Input: part model. Units: mm. Frame: model coordinates. Coordinates: 2 decimals unless noted, no trailing zeros. Write each loop counter-clockwise with the first axis right and the second up, starting at its lowest first coordinate (ties: lowest second). Pieces come first, ordered by that corner, then holes. Notation, with made-up numbers: (27, -23) - (86, -23) arc R22 cw to (86, 0) - close; hole circle Ø6 at (30, 2.25). An arc over 180 degrees is marked (long way). One line per question, with ' | ' between items. Start each with the question number.
1) First-contact query: P1, Ø0.9, axis at y = 15.5, z = 1, coming from the +X side; P2, Ø0.9, axis at y = 27.5, z = 2, coming from the +X side; P3, Ø1.5, axis at y = 25, z = 2, coming from the -X side. Flat tips, straight axial feed; report the tip coordinate or a pass-through.
2) Section query A-A on y = 68.5. Return loops of the section in (x, z), and give its area (3 significant figures).
3) Draft query along X for faces 1 (the cylindrical face through (182.45, 72.19, 1.48)), 2 (the flat face through (140, 15, 0)), 3 (the cylindrical face through (196.41, 57.77, 1.48)). Return one class per face: released by +X, released by -X, zero draft, split by the parting line, or undercut.
4) Section query C-C on x = 105. Return loops of the section in (y, z), and give its area (3 significant figures).
5) Line query: line 1 (Y direction, x = 228.5, z = 0.55); line 2 (Y direction, x = 166.5, z = 1.1); line 3 (X direction, y = 15.5, z = 1.4). Output: solid intervals per line, ascending.
6) Section query D-D on y = 58.5. Return loops of the section in (x, z), and give its area (3 significant figures).
7) Section query B-B on z = 1.15. Return loops of the section in (x, y), and give its area (3 significant figures).
```python
from build123d import *

# Parameters (mm, degrees)
EXTRUDE_1_DEPTH = 3


with BuildPart() as part:
    # Эскиз2 → Бобышка-Вытянуть1 (new body)
    with BuildSketch(Plane.XY):
        with BuildLine():
            Line((0, 0), (172, 0))
            Line((172, 0), (172, 6))
            Line((172, 6), (177, 6))
            Line((177, 6), (177, 0))
            Line((177, 0), (244, 0))
            Line((244, 0), (244, 6))
            Line((244, 6), (250, 6))
            Line((250, 6), (250, 12))
            Line((250, 12), (244, 12))
            Line((244, 12), (214, 12))
            Line((214, 12), (214, 20))
            Line((214, 20), (187, 20))
            Line((187, 20), (187, 32))
            ThreePointArc((187, 32), (196.668498224, 58.076809621), (221, 71.547439867))
            Line((221, 71.547439867), (231, 71.547439867))
            Line((231, 71.547439867), (231, 51.547439867))
            Line((231, 51.547439867), (241, 51.547439867))
            Line((241, 51.547439867), (241, 83.547439867))
            ThreePointArc((241, 83.547439867), (238.656854249, 89.204294116), (233, 91.547439867))
            Line((233, 91.547439867), (219.644566271, 91.547439867))
            ThreePointArc((219.644566271, 91.547439867), (182.048214587, 71.740873017), (167, 32))
            Line((167, 32), (167, 20))
            Line((167, 20), (0, 20))
            Line((0, 20), (-6, 20))
            Line((-6, 20), (-6, 14))
            Line((-6, 14), (0, 14))
            Line((0, 14), (0, 6))
            Line((0, 6), (-6, 6))
            Line((-6, 6), (-6, 0))
            Line((-6, 0), (0, 0))
        make_face()
    extrude(amount=EXTRUDE_1_DEPTH)


solid = part.part
```
Answer key:
1) P1: x = 214 | P2: x = 187 | P3: x = 167
2) outline: (179.38, 0) - (210.64, 0) - (210.64, 3) - (179.38, 3) - close; (231, 0) - (241, 0) - (241, 3) - (231, 3) - close | area: 124 mm²
3) face 1: released by -X | face 2: zero draft | face 3: undercut
4) outline: (0, 0) - (20, 0) - (20, 3) - (0, 3) - close | area: 60.0 mm²
5) line 1: 0 to 12, 71.55 to 91.55 | line 2: 0 to 20 | line 3: -6 to 214
6) outline: (173.17, 0) - (197.04, 0) - (197.04, 3) - (173.17, 3) - close; (231, 0) - (241, 0) - (241, 3) - (231, 3) - close | area: 102 mm²
7) outline: (-6, 0) - (172, 0) - (172, 6) - (177, 6) - (177, 0) - (244, 0) - (244, 6) - (250, 6) - (250, 12) - (214, 12) - (214, 20) - (187, 20) - (187, 32) arc R40 cw to (221, 71.55) - (231, 71.55) - (231, 51.55) - (241, 51.55) - (241, 83.55) arc R8 ccw to (233, 91.55) - (219.64, 91.55) arc R60 ccw to (167, 32) - (167, 20) - (-6, 20) - (-6, 14) - (0, 14) - (0, 6) - (-6, 6) - close | area: 6,990 mm²
